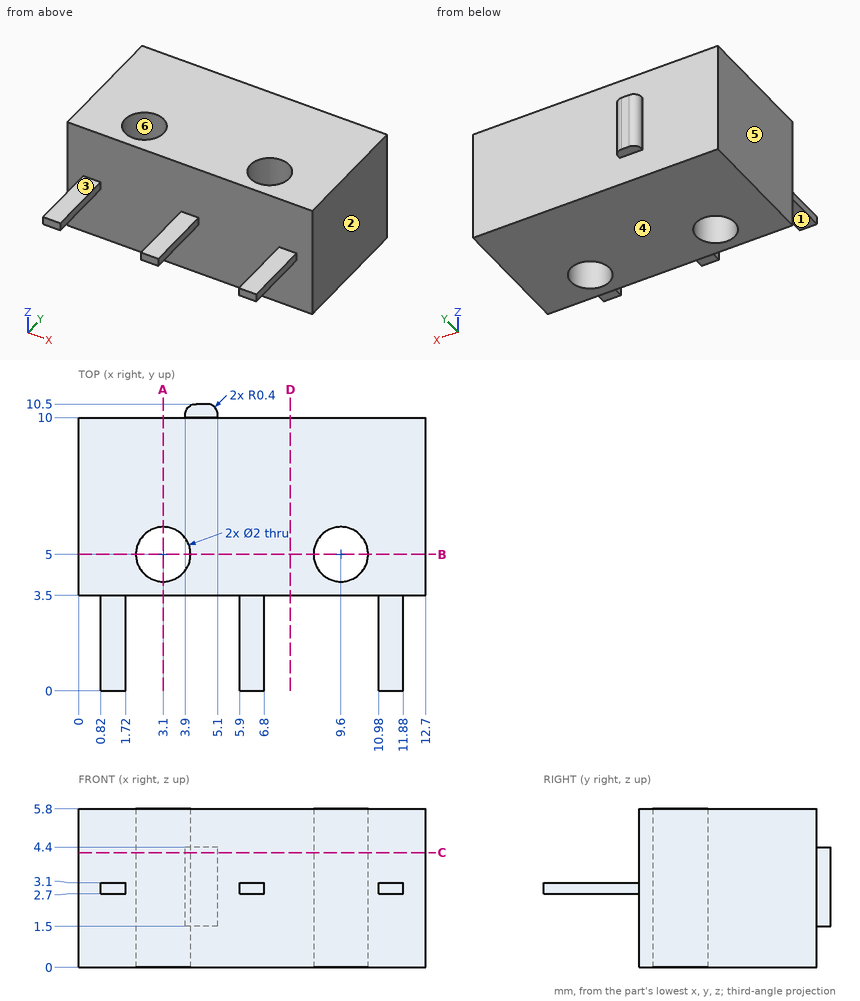
Could you check a few things on this drawing? It's one solid part, dimensions in mm from its lowest x, y, z. A direction names the side the tool comes from. Give positions to 0.01 mm unless a question says otherwise; leave off trailing zeros. Order: outer loops, then holes, each group sorted by start corner. A loop starts at its lowest first (then second) coordinate and runs counter-clockwise, first axis right, second up. Notation, with made-up numbers: (84.25, -34) -> (139.25, -34) arc R23 cw to (139.25, 2) -> close; hole circle Ø3 at (46, 13.25). An arc over 180 degrees is marked (long way). Use CSV: the item, a comma, the result in double quotes. Start each with the question number.
Item 1: Thinking about a two-plate mould opening in X: for the marked faces 4, 5 and 6, which applies, pulls with the +X half, pulls with the -X half, needs draft (parallel to the pull), parting line crosses it, or undercut?
Item 2: Suppose I cut it at A-A (x = 3.1). List the corners of the cut face in (y, z) for me.
Item 3: On a 3-axis mill with a long thin cutter (end or side, diameter ignored), from which of +Z, -Z, +X, -X, +Y, -Y can I reach the whole of each face in a straight line? I mean the marked faces 1, 2 and 3. Say none if no direction works.
Item 4: Suppose I cut it at C-C (z = 4.2). List the corners of the cut face in (x, y) for me.
Item 5: Suppose I cut it at B-B (y = 5). List the corners of the cut face in (x, z) for me.
Item 6: Suppose I cut it at D-D (x = 7.75). List the corners of the cut face in (y, z) for me, and give its area (3 significant figures).
Item 7: I'm going to push flat-ended pins straight in: P1, Ø1.5, axis at x = 8.5, z = 1.5, coming from the -Y side; P2, Ø0.7, axis at x = 6, y = 2.5, coming from the -Z side. Where does each tip first touch, or does it pass through?
Item 8: If I drill on probe 1 along X at (y, z) = (1.5, 2.95); probe 2 along Y at (x, z) = (3.1, 2.4); probe 3 along Y at (x, z) = (8.5, 3.55), over which ranges is the centre line in solid material (lowest first)? Write a range as [from, to].
Answer block:
1,face 4,"needs draft"
1,face 5,"pulls with the -X half"
1,face 6,"undercut"
2,outline,"(3.5, 0) -> (4, 0) -> (4, 5.8) -> (3.5, 5.8) -> close; (6, 0) -> (10, 0) -> (10, 5.8) -> (6, 5.8) -> close"
3,face 1,"-Z, +X, -X, -Y"
3,face 2,"+Z, -Z, +X, +Y, -Y"
3,face 3,"+Z, +X, -X, -Y"
4,outline,"(0, 3.5) -> (12.7, 3.5) -> (12.7, 10) -> (5.1, 10) -> (5.1, 10.1) arc R0.4 ccw to (4.7, 10.5) -> (4.3, 10.5) arc R0.4 ccw to (3.9, 10.1) -> (3.9, 10) -> (0, 10) -> close; hole circle Ø2 at (3.1, 5); hole circle Ø2 at (9.6, 5)"
5,outline,"(0, 0) -> (2.1, 0) -> (2.1, 5.8) -> (0, 5.8) -> close; (4.1, 0) -> (8.6, 0) -> (8.6, 5.8) -> (4.1, 5.8) -> close; (10.6, 0) -> (12.7, 0) -> (12.7, 5.8) -> (10.6, 5.8) -> close"
6,outline,"(3.5, 0) -> (10, 0) -> (10, 5.8) -> (3.5, 5.8) -> close"
6,area,"37.7 mm^2"
7,P1,"stops at y = 3.5"
7,P2,"stops at z = 2.7"
8,probe 1,"x = [0.82, 1.72], [5.9, 6.8], [10.98, 11.88]"
8,probe 2,"y = [3.5, 4], [6, 10]"
8,probe 3,"y = [3.5, 10]"
